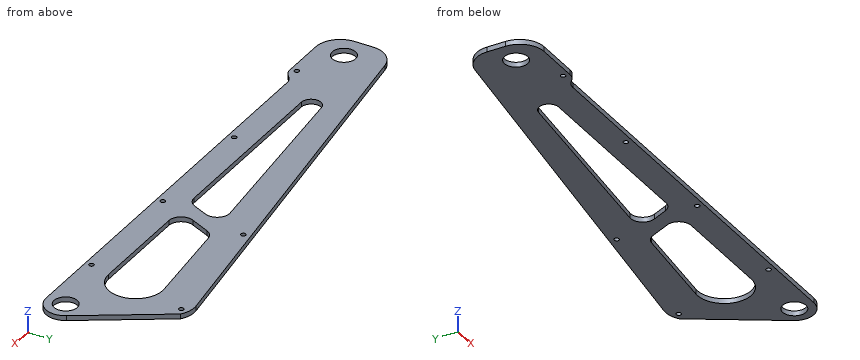
from build123d import *

# Parameters (mm, degrees)
SKETCH_1_R      = 2
SKETCH_1_R_2    = 9.52
EXTRUDE_1_DEPTH = 4


with BuildPart() as part:
    # 草图1 → 凸台-拉伸1 (new body)
    with BuildSketch(Plane.XY):
        with BuildLine():
            Line((-217.492033448, 3.233624406), (131.287449442, 52.251384058))
            ThreePointArc((131.287449442, 52.251384058), (139.247292364, 51.764539209), (146.384140968, 48.206237756))
            Line((146.384140968, 48.206237756), (188.878227524, -20.121950331))
            ThreePointArc((188.878227524, -20.121950331), (189.277074538, -36.343590473), (175.291428571, -44.571736969))
            Line((175.291428571, -44.571736969), (-162.726593938, -44.571736969))
            ThreePointArc((-162.726593938, -44.571736969), (-166.146795371, -45.174810761), (-169.154470035, -46.911292538))
            Line((-169.154470035, -46.911292538), (-171.920397674, -49.2321814))
            ThreePointArc((-171.920397674, -49.2321814), (-174.928072338, -50.968663177), (-178.348273771, -51.571736969))
            Line((-178.348273771, -51.571736969), (-214.708571429, -51.571736969))
            ThreePointArc((-214.708571429, -51.571736969), (-228.850707052, -45.713872593), (-234.708571429, -31.571736969))
            Line((-234.708571429, -31.571736969), (-234.708571429, -16.571736969))
            ThreePointArc((-234.708571429, -16.571736969), (-229.802763033, -3.450556389), (-217.492033448, 3.233624406))
        make_face()
        with Locations((120.291428571, -39.571736969)):
            Circle(SKETCH_1_R, mode=Mode.SUBTRACT)
        with Locations((31.062311574, 32.428263031)):
            Circle(SKETCH_1_R, mode=Mode.SUBTRACT)
        with Locations((175.291428571, -28.571736969)):
            Circle(SKETCH_1_R_2, mode=Mode.SUBTRACT)
        with Locations((-79.708571429, -39.571736969)):
            Circle(SKETCH_1_R, mode=Mode.SUBTRACT)
        with Locations((-214.708571429, -28.571736969)):
            Circle(SKETCH_1_R_2, mode=Mode.SUBTRACT)
        with Locations((140.291428571, 45.428263031)):
            Circle(SKETCH_1_R, mode=Mode.SUBTRACT)
        with Locations((-179.708571429, -46.571736969)):
            Circle(SKETCH_1_R, mode=Mode.SUBTRACT)
        with Locations((20.291428571, -39.571736969)):
            Circle(SKETCH_1_R, mode=Mode.SUBTRACT)
        with BuildLine():
            Line((40.988284343, -22.571736969), (125.291428571, -22.571736969))
            ThreePointArc((125.291428571, -22.571736969), (147.261913315, 0.567473351), (123.016064666, 21.310281199))
            Line((123.016064666, 21.310281199), (47.451409263, 13.452820882))
            ThreePointArc((47.451409263, 13.452820882), (42.683150544, 11.650822458), (39.422587713, 7.732631605))
            Line((39.422587713, 7.732631605), (31.925206472, -8.345554352))
            ThreePointArc((31.925206472, -8.345554352), (32.554369884, -17.944733053), (40.988284343, -22.571736969))
        make_face(mode=Mode.SUBTRACT)
        with BuildLine():
            Line((-144.708571429, -22.571736969), (5.680190936, -22.571736969))
            ThreePointArc((5.680190936, -22.571736969), (11.053187019, -21.005651427), (14.743268806, -16.797919586))
            Line((14.743268806, -16.797919586), (20.441380932, -4.578278698))
            ThreePointArc((20.441380932, -4.578278698), (19.522676532, 5.450418959), (10.344046742, 9.594275814))
            Line((10.344046742, 9.594275814), (-145.535976485, -6.614639453))
            ThreePointArc((-145.535976485, -6.614639453), (-152.697838608, -14.985995267), (-144.708571429, -22.571736969))
        make_face(mode=Mode.SUBTRACT)
    extrude(amount=EXTRUDE_1_DEPTH)


solid = part.part
For this review, take the finished solid that the model builds, in its own axes (mm). Give positions to 0.01 mm unless a question says otherwise; leave off trailing zeros. Order: outer loops, then holes, each group sorted by start corner. A loop starts at its lowest first (then second) coordinate and runs counter-clockwise, first axis right, second up. Notation, with made-up numbers: (-9.75, 20) - (11.25, 20) arc R11 cw to (11.25, 26) - close; hole circle Ø7 at (59.25, 31.5). An arc over 180 degrees is marked (long way). Answer as a JSON object with one key per item and string values. Group by question number.
Item 1: Take a section at B-B on z = 0.7. Give the number of separate pieces and of enclosed holes in the cut face, and give its area (3 significant figures).
Item 2: Clearance check with flat-ended pins moving along their axes: pin 1 Ø3.5 at (x, y) = (20.29, -39.57) entering from +Z; pin 2 Ø2 at (x, z) = (75, 3) entering from +Y; pin 3 Ø2 at (x, z) = (44.5, 2.5) entering from +Y; pin 4 Ø1.2 at (x, z) = (88, 1.5) entering from -Y. State where each tip first meets the part, or that it passes through.
Item 3: Take a section at A-A on x = -58.5. Give the boundary of the cut face in (y, z), and give its area (3 significant figures).
Item 4: Wall thickness on line 1 along X through (y, z) = (-29.5, 0.35); line 2 along X through (y, z) = (-18.5, 2.25); line 3 along Y through (x, z) = (142, 2.2): over which ranges is each line inside the solid? List them lowest first.
Item 5: Take a section at C-C on x = 51.5. Give the boundary of the cut face in (y, z).
Reported:
{
 "1": {"separate pieces": "1", "enclosed holes": "10", "area": "21,200 mm^2"},
 "2": {"pin 1": "through", "pin 2": "y = 44.48", "pin 3": "y = 40.19", "pin 4": "y = -44.57"},
 "3": {"outline": "(-44.57, 0) - (-22.57, 0) - (-22.57, 4) - (-44.57, 4) - close; (2.44, 0) - (25.58, 0) - (25.58, 4) - (2.44, 4) - close", "area": "181 mm^2"},
 "4": {"line 1": "-234.71 to -224.18, -205.23 to 165.82, 184.77 to 191.26", "line 2": "-234.71 to -151.68, 13.73 to 32.93, 138.04 to 187.87", "line 3": "-44.57 to -14.88, 13.74 to 44.39, 46.47 to 50.81"},
 "5": {"outline": "(-44.57, 0) - (-22.57, 0) - (-22.57, 4) - (-44.57, 4) - close; (13.87, 0) - (41.04, 0) - (41.04, 4) - (13.87, 4) - close"}
}
